Geometry: final body of the model. Coordinates: model frame, mm. A direction names the side the tool comes from. Round coordinates to 2 decimals unless told otherwise and drop trailing zeros. Loops run counter-clockwise (first coordinate to the right, second up) from the corner with the lowest first, then second, coordinate; pieces in that order, holes last. Notation, with made-up numbers: (-1.75, -8) - (29.25, -8) arc R14 cw to (29.25, 5) - close; hole circle Ø6 at (-2, 18). An arc over 180 degrees is marked (long way). Write item = value, one per line. Start each with the question number.
Item 1: Section D-D (y = 6.5). Return loops of the section in (x, z).
Item 2: Line query: line 1 (Z direction, x = 7.75, y = 15); line 2 (Y direction, x = 7.75, z = 19); line 3 (Z direction, x = 7, y = -6). Output: solid intervals per line, ascending. Write a range as from..to.
Item 3: Section C-C (x = 1.25). Return loops of the section in (y, z).
Item 4: Draft query along Z for faces 4 (the flat face through (5, -30, -25)), 5 (the cylindrical face through (5.1, 11.8, 5.6)), 6 (the flat face through (5, -40.011, 0)), 7 (the flat face through (5, -30, 25)). Return one class per face: pulls with the +Z half, pulls with the -Z half, needs draft (parallel to the pull), parting line crosses it, or undercut.
Item 5: Section B-B (y = 15). Return loops of the section in (x, z), plus the area to 3 significant figures.
Item 6: Section A-A (z = 8). Return loops of the section in (x, y).
Item 7: Access query for faces 1 (the flat face through (5, 29.989, 0)), 2 (the flat face through (5, -20.011, 20)), 3 (the flat face through (5, 5, -15)). Directions: +Z, -Z, +X, -X, +Y, -Y. A direction counts if a zero-diameter tool reaches every point of the face in a straight line with its end or side. Return the directions, or none.
Item 8: First-contact query: pin 1 (1.5 mm diameter, centred on x = 8.5, z = 16, fed in from +Y); pin 2 (1.5 mm diameter, centred on x = 5, y = -5.5, fed in from -Z); pin 3 (3 mm diameter, centred on x = 5, y = 11, fed in from +Z). Flat tips, straight axial feed; report the tip coordinate or a pass-through.
from build123d import *

# Parameters (mm, degrees)
PAD_DEPTH    = 10
SKETCH001_R  = 4
POCKET_DEPTH = 10


with BuildPart() as part:
    # Sketch → Pad (new body)
    with BuildSketch(Plane.YZ):
        Polygon((-40.011498, 25), (-20.011498, 25), (-20.011498, 15), (29.988502, 15), (29.988502, -15), (-20.011498, -15), (-20.011498, -25), (-40.011498, -25), align=None)
    extrude(amount=PAD_DEPTH)

    # Sketch001 → Pocket (cut)
    with BuildSketch(Plane.YZ.offset(10)):
        with Locations((15, 8)):
            Circle(SKETCH001_R)
        with Locations((15, -8)):
            Circle(SKETCH001_R)
    extrude(amount=-POCKET_DEPTH, mode=Mode.SUBTRACT)


solid = part.part
Taken from the geometry:
q1.outline = (0, -15) - (10, -15) - (10, 15) - (0, 15) - close
q2.line_1 = -15..-12, -4..4, 12..15
q2.line_2 = -40.01..-20.01
q2.line_3 = -15..15
q3.outline = (-40.01, -25) - (-20.01, -25) - (-20.01, -15) - (29.99, -15) - (29.99, 15) - (-20.01, 15) - (-20.01, 25) - (-40.01, 25) - close; hole circle Ø8 at (15, -8); hole circle Ø8 at (15, 8)
q4.face_4 = pulls with the -Z half
q4.face_5 = undercut
q4.face_6 = needs draft
q4.face_7 = pulls with the +Z half
q5.outline = (0, -15) - (10, -15) - (10, -12) - (0, -12) - close; (0, -4) - (10, -4) - (10, 4) - (0, 4) - close; (0, 12) - (10, 12) - (10, 15) - (0, 15) - close
q5.area = 140 mm^2
q6.outline = (0, -40.01) - (10, -40.01) - (10, 11) - (0, 11) - close; (0, 19) - (10, 19) - (10, 29.99) - (0, 29.99) - close
q7.face_1 = +Z, -Z, +X, -X, +Y
q7.face_2 = +Z, +X, -X, +Y
q7.face_3 = -Z, +X, -X, +Y
q8.pin_1 = -20.01
q8.pin_2 = -15
q8.pin_3 = 15
